Verification items for the finished model (mm, model axes). A direction names the side the tool comes from. Round coordinates to 2 decimals unless told otherwise and drop trailing zeros. Loops run counter-clockwise (first coordinate to the right, second up) from the corner with the lowest first, then second, coordinate; pieces in that order, holes last. Notation, with made-up numbers: M 7,-29 L 38,-29 A14 cw 38,-16 Z; hole C -6,50.25 d9. An arc over 180 degrees is marked long. One line per item, written item: value.
from build123d import *

# Parameters (mm, degrees)
SKETCH1_R           = 1.5
BOSS_EXTRUDE1_DEPTH = 5


with BuildPart() as part:
    # Sketch1 → Boss-Extrude1 (new body)
    # profile 1 of 2: a face of its own
    with BuildSketch(Plane.XY):
        Polygon((-30, -45.891400943), (-30, -50.891400943), (-35, -50.891400943), (-35, -80.891400943), (-30, -80.891400943), (-30, -85.891400943), (-14, -85.891400943), (-10, -85.891400943), (-10, -90.891400943), (20, -90.891400943), (20, -85.891400943), (85, -85.891400943), (110, -85.891400943), (115, -85.891400943), (140, -85.891400943), (140, -80.891400943), (145, -80.891400943), (145, -50.891400943), (140, -50.891400943), (140, -45.891400943), (115, -45.891400943), (115, -40.891400943), (75, -40.891400943), (75, -45.891400943), (35, -45.891400943), (35, -40.891400943), (-5, -40.891400943), (-5, -45.891400943), align=None)
        with Locations((-8.25, -73.391400943)):
            Circle(SKETCH1_R, mode=Mode.SUBTRACT)
        with BuildLine():
            ThreePointArc((3.5, -73.391400943), (2.474873734, -75.866274677), (0, -76.891400943))
            ThreePointArc((0, -76.891400943), (-2.474873734, -75.866274677), (-3.5, -73.391400943))
            ThreePointArc((-3.5, -73.391400943), (0, -69.891400943), (3.5, -73.391400943))
        make_face(mode=Mode.SUBTRACT)
        with BuildLine():
            ThreePointArc((9.75, -73.391400943), (8.25, -74.891400943), (6.75, -73.391400943))
            ThreePointArc((6.75, -73.391400943), (8.25, -71.891400943), (9.75, -73.391400943))
        make_face(mode=Mode.SUBTRACT)
        with Locations((101.75, -73.391400943)):
            Circle(SKETCH1_R, mode=Mode.SUBTRACT)
        with BuildLine():
            ThreePointArc((113.5, -73.391400943), (112.474873734, -75.866274677), (110, -76.891400943))
            ThreePointArc((110, -76.891400943), (107.525126266, -75.866274677), (106.5, -73.391400943))
            ThreePointArc((106.5, -73.391400943), (110, -69.891400943), (113.5, -73.391400943))
        make_face(mode=Mode.SUBTRACT)
        with BuildLine():
            ThreePointArc((119.75, -73.391400943), (118.25, -74.891400943), (116.75, -73.391400943))
            ThreePointArc((116.75, -73.391400943), (118.25, -71.891400943), (119.75, -73.391400943))
        make_face(mode=Mode.SUBTRACT)
    # profile 2 of 2: a face of its own
    with BuildSketch(Plane.XY):
        Polygon((110, -85.891400943), (85, -85.891400943), (85, -90.891400943), (115, -90.891400943), (115, -85.891400943), align=None)
    extrude(amount=BOSS_EXTRUDE1_DEPTH)


solid = part.part
(1) Thickness scan on L1, parallel to Y at x = -8.25, z = 1.9; L2, parallel to Y at x = 101.75, z = 3; L3, parallel to Y at x = 77, z = 1.65. Record the ranges inside material, lowest first. Write a range as from..to.
Completed:
L1: y = -90.89..-74.89, -71.89..-45.89
L2: y = -90.89..-74.89, -71.89..-40.89
L3: y = -85.89..-40.89
(2) Sectioned sample at C-C on z = 1.35. Count the separate pieces of the cut face and the enclosed holes in it, and give its area (3 significant figures).
Completed:
separate pieces: 1
enclosed holes: 6
area: 7,690 mm^2
(3) Mould release check, pull along Y, two halves, no side actions. Record for faces 1 (the face through (115, -88, 2)), 2 (the face through (52, -85.891, 2)), 3 (the face through (102.56, -72.13, 2.46)), 4 (the face through (128, -45.891, 2)): +Y half, -Y half, draft (parallel to the pull), parting line (faces both ways), or undercut.
Completed:
face 1: draft
face 2: -Y half
face 3: undercut
face 4: +Y half
(4) Sectioned sample at B-B on x = 118.25. Enter the section's corners in (y, z).
Completed:
outline: M -85.89,0 L -74.89,0 L -74.89,5 L -85.89,5 Z; M -71.89,0 L -45.89,0 L -45.89,5 L -71.89,5 Z
(5) Tool access check on faces 5 (the face through (75, -43, 2)), 6 (the face through (143, -50.891, 2)), 7 (the face through (-30, -48, 2)), 8 (the face through (20, -88, 2)). Record the directions out of +Z, -Z, +X, -X, +Y, -Y that give a thin tool (end or side, any length) a straight path to the whole face; none if there is none.
Completed:
face 5: +Z, -Z, +Y
face 6: +Z, -Z, +X, +Y
face 7: +Z, -Z, -X, +Y
face 8: +Z, -Z, -Y
(6) Depth check by flat-ended pin: pin 1 Ø2.5 at (y, z) = (-83.5, 1.5) entering from -X; pin 2 Ø2.5 at (y, z) = (-42.5, 3) entering from +X; pin 3 Ø2.5 at (x, z) = (-17.5, 1.5) entering from -Y. Enter the tip coordinate at first touch or a pass-through.
Completed:
pin 1: stops at x = -30
pin 2: stops at x = 115
pin 3: stops at y = -85.89
(7) Sectioned sample at A-A on x = -8.25. Enter the section's corners in (y, z), and give its area (3 significant figures).
Completed:
outline: M -90.89,0 L -74.89,0 L -74.89,5 L -90.89,5 Z; M -71.89,0 L -45.89,0 L -45.89,5 L -71.89,5 Z
area: 210 mm^2
